Autodesk Fusion 360 part; units mm, degrees
sketch "Outer" plane through (0, 0, 0) normal (0, 1, 0) x (1, 0, 0)
  circle A0 centre (0, 0) radius 11
  dimension "d1" = 22
extrude "Extrude1" add sketch "Outer" along normal blind 20
sketch "Inner" plane through (0, 20, 0) normal (0, 1, 0) x (-1, 0, 0)
  circle A0 centre (0, 0) radius 11
  circle A1 centre (0, 0) radius 9
  dimension "d4" = 18
extrude "Extrude2" cut sketch "Inner" against normal blind 18 contours A1
sketch "Shaft" plane through (0, 2, 0) normal (0, 1, 0) x (-1, 0, 0)
  circle A0 centre (0, 0) radius 9
  line L0 (-1.7, 2.7111) -> (-1.7, -2.7111)
  arc A1 (-1.7, -2.7111) -> (-1.7, 2.7111) centre (0, 0) ccw
  arc A2 (-3.7, -3.6538) -> (-3.7, 3.6538) centre (0, 0) ccw
  line L1 (-3.7, 3.6538) -> (-3.7, -3.6538)
  dimension "d7" = 6.4
  dimension "d8" = 1.7
  dimension "d9" = 2
extrude "Extrude3" add sketch "Shaft" along normal blind 12.5 contours A2 L1
extrude "Extrude4" add 1 faces at (0.0662, 2, 0.598) along direction (0, 1, 0) blind 5
equation "d5 = -( 20 mm - 2 mm )"
equation "d7 = 6 mm + 0.2 mm + 0.2 mm"
equation "d8 = ( 4.5 mm - 3 mm ) + 0.2 mm"
equation "d10 = 20 mm - 2 mm - 5.5 mm"
equation "d12 = 20 mm - 2 mm - 5.5 mm - 7.5 mm"
Read the model definition and answer for the solid it produces. Units are mm, in the model's axes. A direction names the side the tool comes from. Coordinates: 2 decimals unless noted, no trailing zeros. Write each loop counter-clockwise with the first axis right and the second up, starting at its lowest first coordinate (ties: lowest second). Pieces come first, ordered by that corner, then holes. Notation, with made-up numbers: (26, -15) - (65, -15) arc R7 cw to (65, -7) - close; hole circle Ø7 at (81.25, 35.25). An arc over 180 degrees is marked (long way). One line per question, with ' | ' between items.
Q1. Find section A-A, the plane y = 10.75. Write down the section's boundary in (x, z), plus the area to 3 significant figures.
Result set:
outline: circle Ø22 at (0, 0); (3.7, -3.65) - (3.7, 3.65) arc R5.2 ccw (long way) to start; hole circle Ø18 at (0, 0); hole (1.7, -2.71) - (1.7, 2.71) arc R3.2 ccw (long way) to start | area: 177 mm^2
Q2. Each of these flat-tipped pins is pushed along its axis until it touches: P1, Ø4.5, axis at x = 0, z = -1.5, coming from the +Y side; P2, Ø3, axis at x = -4, y = 15, coming from the -Z side. Where does it stop, or does it pass through?
Result set:
P1: y = 14.5 | P2: z = -10.71
Q3. For faces 1 (the cylindrical face through (1.172, 11.126, 8.923)), 2 (the flat face through (0, 0, 0)), determine the directions among +Z, -Z, +X, -X, +Y, -Y from which every point of the face is accessible in a straight line to the end or side of a thin tool.
Result set:
face 1: +Y | face 2: +Z, -Z, +X, -X, -Y
Q4. Determine the mould class of faces 3 (the flat face through (2, 20, 9)), 4 (the cylindrical face through (-2.38, 9.86, -10.74)), 5 (the flat face through (4, 2, 0)) for opening direction X: +X half, -X half, draft (parallel to the pull), parting line (faces both ways), or undercut.
Result set:
face 3: draft | face 4: parting line | face 5: undercut
Q5. Find section C-C, the plane x = 0. Write down the section's boundary in (y, z).
Result set:
outline: (0, -11) - (20, -11) - (20, -9) - (2, -9) - (2, -5.2) - (14.5, -5.2) - (14.5, -3.2) - (7, -3.2) - (7, 3.2) - (14.5, 3.2) - (14.5, 5.2) - (2, 5.2) - (2, 9) - (20, 9) - (20, 11) - (0, 11) - close
Q6. Find section D-D, the plane y = 5. Write down the section's boundary in (x, z).
Result set:
outline: circle Ø22 at (0, 0); (3.7, -3.65) - (3.7, 3.65) arc R5.2 ccw (long way) to start; hole circle Ø18 at (0, 0)
Q7. Consider L1, parallel to Z at x = 0, y = 12.5; L2, parallel to Z at x = -2.75, y = 12; L3, parallel to X at y = 11.25, z = -4.5. Determine where each line is inside the solid, lowest interval first. Write a range as [from, to].
Result set:
L1: [-11, -9], [-5.2, -3.2], [3.2, 5.2], [9, 11] | L2: [-10.65, -8.57], [-4.41, -1.64], [1.64, 4.41], [8.57, 10.65] | L3: [-10.04, -7.79], [-2.61, 2.61], [7.79, 10.04]
Q8. Find section B-B, the plane z = 0. Write down the section's boundary in (x, y).
Result set:
outline: (-11, 0) - (11, 0) - (11, 20) - (9, 20) - (9, 2) - (3.7, 2) - (3.7, 14.5) - (1.7, 14.5) - (1.7, 7) - (-3.2, 7) - (-3.2, 14.5) - (-5.2, 14.5) - (-5.2, 2) - (-9, 2) - (-9, 20) - (-11, 20) - close
